For this review, use the dimensioned drawing (mm, ordinates from the lowest corner) and the shaded views. A direction names the side the tool comes from. Round coordinates to 2 decimals unless told otherwise and drop trailing zeros. Order: outer loops, then holes, each group sorted by start corner. A loop starts at its lowest first (then second) coordinate and runs counter-clockwise, first axis right, second up. Notation, with made-up numbers: (-22, 0.5) -> (-15, 0.5) arc R22 ccw to (-15, 11.5) -> close; hole circle Ø4 at (12, 82.5). An arc over 180 degrees is marked (long way). Answer in a Markdown table with one row per item.
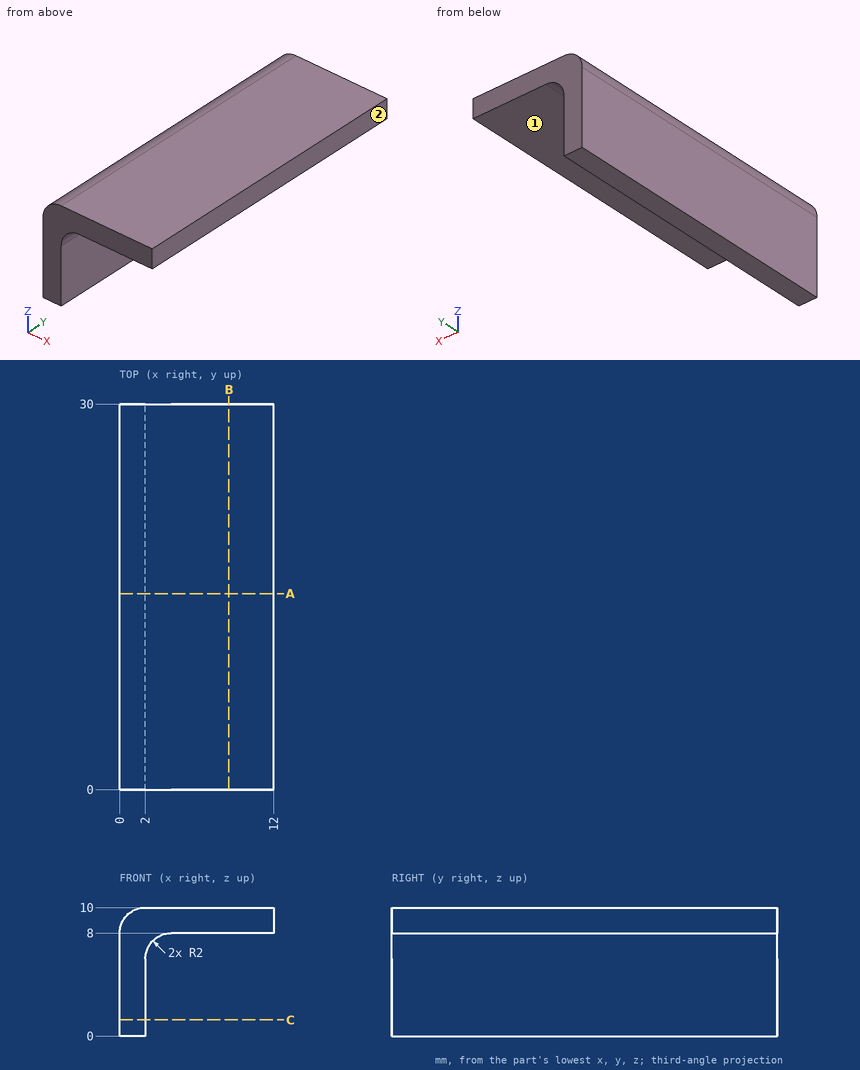
Q1. To check wall thickness, follow probe 1 along Z at (x, y) = (11.25, 15.25); probe 2 along X at (y, z) = (22.5, 6); probe 3 along X at (y, z) = (23, 8.75). State the ranges of each line that lie inside material, in increasing order.
Answer key:
| item | result |
|---|---|
| probe 1 | z = 8 to 10 |
| probe 2 | x = 0 to 2 |
| probe 3 | x = 0.15 to 12 |
Q2. Take a section at A-A, the plane y = 15.25. Write out the cut boundary in (x, z), then the cut area to 3 significant figures.
Answer key:
| item | result |
|---|---|
| outline | (0, 0) -> (2, 0) -> (2, 6) arc R2 cw to (4, 8) -> (12, 8) -> (12, 10) -> (2, 10) arc R2 ccw to (0, 8) -> close |
| area | 40.0 mm^2 |
Q3. Take a section at B-B, the plane x = 8.5. Write out the cut boundary in (y, z), then the cut area to 3 significant figures.
Answer key:
| item | result |
|---|---|
| outline | (0, 8) -> (30, 8) -> (30, 10) -> (0, 10) -> close |
| area | 60.0 mm^2 |
Q4. Take a section at C-C, the plane z = 1.25. Write out the cut boundary in (x, y), then the cut area to 3 significant figures.
Answer key:
| item | result |
|---|---|
| outline | (0, 0) -> (2, 0) -> (2, 30) -> (0, 30) -> close |
| area | 60.0 mm^2 |
Q5. Tool access review of the marked faces 1 and 2: name each direction out of +Z, -Z, +X, -X, +Y, -Y from which nothing blocks a thin tool from reaching the whole face with its end or side.
Answer key:
| item | result |
|---|---|
| face 1 | -Z, +X, +Y, -Y |
| face 2 | +Z, -Z, +X, +Y, -Y |
Q6. Clearance check with flat-ended pins moving along their axes: pin 1 Ø2.5 at (x, y) = (9, 18.5) entering from -Z; pin 2 Ø6 at (y, z) = (8, 6) entering from +X; pin 3 Ø3 at (y, z) = (15, 1.5) entering from +X. State where each tip first meets the part, or that it passes through.
Answer key:
| item | result |
|---|---|
| pin 1 | stops at z = 8 |
| pin 2 | stops at x = 12 |
| pin 3 | stops at x = 2 |
